Can you work these out from the model? Positions are in its coordinate system, mm. A direction names the side the tool comes from. Give positions to 0.01 mm unless a question says otherwise; leave off trailing zeros. Loops run counter-clockwise (first coordinate to the right, second up) from the corner with the lowest first, then second, coordinate; pieces in that order, holes last.
from build123d import *

# Parameters (mm, degrees)
SKETCH1_R           = 12
SKETCH1_R_2         = 3.5
BOSS_EXTRUDE1_DEPTH = 0.5
BOSS_EXTRUDE3_DEPTH = 5


with BuildPart() as part:
    # Sketch1 → Boss-Extrude1 (new body, symmetric)
    with BuildSketch(Plane(origin=(0, 0, 0), x_dir=(1, 0, 0), z_dir=(0, 1, 0))):
        Circle(SKETCH1_R)
        Circle(SKETCH1_R_2, mode=Mode.SUBTRACT)
    extrude(amount=BOSS_EXTRUDE1_DEPTH, both=True)

    # Sketch5 → Boss-Extrude3 (add)
    with BuildSketch(Plane(origin=(0, 0.5, 0), x_dir=(1, 0, 0), z_dir=(0, 1, 0))):
        Polygon((-6.491303756, -4.950065272), (-2.866072607, -6.640538319), (-3.5, -8), (-7.125231148, -6.309526953), align=None)
        Polygon((7.125231148, -6.309526953), (6.491303756, -4.950065272), (2.866072607, -6.640538319), (3.5, -8), align=None)
    extrude(amount=BOSS_EXTRUDE3_DEPTH)


solid = part.part
(1) Will this pin go through, and if not, where does the flat tip stop? P1, Ø2, axis at x = 2, y = 2.5, coming from the -Z side.
Returned:
P1: stops at z = 6.58
(2) Please list where these lines run through material, in increasing order: probe 1 along X at (y, z) = (0, 0); probe 2 along Y at (x, z) = (-9, 0).
Returned:
probe 1: x = -12 to -3.5, 3.5 to 12
probe 2: y = -0.5 to 0.5
(3) Which directions (+Z, -Z, +X, -X, +Y, -Y) give clear straight access to the entire face, cutting with the end or side of a thin tool? Please do faces 4 (the flat face through (6.813, 2.965, 5.639)), 5 (the flat face through (-6.813, 2.965, 5.639)), 6 (the flat face through (-5.287, 2.965, 7.167)), 7 (the flat face through (-4.704, 2.965, 5.783)).
Returned:
face 4: -Z, +X, +Y
face 5: -Z, -X, +Y
face 6: +Z, -X, +Y
face 7: -Z, +Y
(4) Thinking about a two-plate mould opening in X: for faces 1 (the flat face through (5.287, 2.965, 7.167)), 2 (the flat face through (-5, 5.5, 6)), 3 (the flat face through (-3.18, 2.96, 7.31)), which applies, pulls with the +X half, pulls with the -X half, needs draft (parallel to the pull), parting line crosses it, or undercut?
Returned:
face 1: pulls with the +X half
face 2: needs draft
face 3: undercut
(5) Suppose I cut it at C-C on x = 4.5. List the corners of the cut face in (y, z) for me, plus the area to 3 significant figures.
Returned:
outline: (-0.5, -11.12) - (0.5, -11.12) - (0.5, 5.88) - (5.5, 5.88) - (5.5, 7.53) - (0.5, 7.53) - (0.5, 11.12) - (-0.5, 11.12) - close
area: 30.5 mm2
(6) Suppose I cut it at A-A on z = 0. List the corners of the cut face in (x, y) for me.
Returned:
outline: (-12, -0.5) - (-3.5, -0.5) - (-3.5, 0.5) - (-12, 0.5) - close; (3.5, -0.5) - (12, -0.5) - (12, 0.5) - (3.5, 0.5) - close
(7) Suppose I cut it at B-B on x = 0. List the corners of the cut face in (y, z) for me, plus the area to 3 significant figures.
Returned:
outline: (-0.5, -12) - (0.5, -12) - (0.5, -3.5) - (-0.5, -3.5) - close; (-0.5, 3.5) - (0.5, 3.5) - (0.5, 12) - (-0.5, 12) - close
area: 17.0 mm2
(8) Suppose I cut it at D-D on z = -9. List the corners of the cut face in (x, y) for me.
Returned:
outline: (-7.94, -0.5) - (7.94, -0.5) - (7.94, 0.5) - (-7.94, 0.5) - close
